The listing builds one solid part. Answer for the finished solid, in the listing's coordinates (mm). A direction names the side the tool comes from. Give positions to 0.01 mm unless a question says otherwise; leave off trailing zeros. Loops run counter-clockwise (first coordinate to the right, second up) from the corner with the lowest first, then second, coordinate; pieces in that order, holes last. Notation, with made-up numbers: (2.25, 27) - (53.25, 27) arc R27 ccw to (53.25, 44) - close; hole circle Ø1 at (38, 38). An arc over 180 degrees is marked (long way). Answer as CSV lines item,"result". Start each with the question number.
1) A cutting plane is placed at D-D (x = -38.5). Determine the outline of the cut face in (y, z), and give its area (3 significant figures).
2) For a pull along X with two mould halves and no side action, classify faces 4 (the face through (51.598, 9.86, 189.239)), 5 (the face through (-2, 0, 99)), 6 (the face through (0, 10, 105)), 7 (the face through (130, 296, 128)) as pulls with the +X half, pulls with the -X half, needs draft (parallel to the pull), parting line crosses it, or undercut.
3) A cutting plane is placed at C-C (x = 32). Determine the outline of the cut face in (y, z) (3 decimals), and give its area (3 significant figures).
4) A cutting plane is placed at B-B (z = 76). Determine the outline of the cut face in (x, y), and give its area (3 significant figures).
5) For faces 1 (the face through (-25, 280, 124)), 2 (the face through (-52.407, 9.86, 191.193)), 3 (the face through (2, 600, 99)), determine the directions among +Z, -Z, +X, -X, +Y, -Y from which every point of the face is accessible in a straight line to the end or side of a thin tool.
6) Find the intervals of material crossed by line 1 along Y through (x, z) = (63.5, 99); line 2 along X through (y, z) = (101.5, 236); line 3 along X through (y, z) = (341, 82.5), in increasing order.
7) Flat-ended cylindrical pins translate along their axes: pin 1 (4 mm diameter, centred on x = -68, y = 310.5, fed in from -Z); pin 2 (12 mm diameter, centred on x = 65, y = 374.5, fed in from +Z). Find the tip coordinate at first contact, or state that the pin passes through.
8) A cutting plane is placed at A-A (y = 449). Determine the outline of the cut face in (x, z), and give its area (3 significant figures).
```python
from build123d import *

# Parameters (mm, degrees)
F1_DEPTH = 260
F2_W     = 210
F2_H     = 110
F3_DEPTH = 225
F4_R     = 104.99999
F6_DEPTH = 600.001


# Not quite as in the source:
# - a fillet or chamfer is up to 0.001 mm smaller than in the source, because OpenCascade refuses the exact size


with BuildPart() as f1:
    # F0 (on Top) → F1 (new body)
    with BuildSketch(Plane.XY):
        Polygon((-130, 0), (0, 0), (130, 0), (130, 600), (-130, 600), align=None)
    extrude(amount=F1_DEPTH)

    # F2 (on face) → F3 (cut)
    with BuildSketch(Plane.XY.offset(260)):
        with Locations((0, 525)):
            Rectangle(F2_W, F2_H)
        with Locations((0, 225)):
            Rectangle(F2_W, F2_H)
        with Locations((0, 375)):
            Rectangle(F2_W, F2_H)
        with Locations((0, 75)):
            Rectangle(F2_W, F2_H)
    extrude(amount=-F3_DEPTH, mode=Mode.SUBTRACT)

    # F4 (radius 105 in the source; OpenCascade refuses exactly that, so slightly less here)
    f4_edges = [f1.edges().sort_by_distance(p)[0] for p in [
        (-105, 75, 35),
        (105, 75, 35),
        (-105, 225, 35),
        (-105, 375, 35),
        (-105, 525, 35),
        (105, 225, 35),
        (105, 375, 35),
        (105, 525, 35),
    ]]
    fillet(f4_edges, radius=F4_R)

    # F5 (on face) → F6 (cut, through all)
    with BuildSketch(Plane.XZ):
        with BuildLine():
            ThreePointArc((23.0969883128, 120.4329141909), (24.5196320101, 125.1227419496), (25, 130))
            ThreePointArc((25, 130), (-4.8772580504, 154.5196320101), (-23.0969883128, 120.4329141909))
            ThreePointArc((-23.0969883128, 120.4329141909), (0, 105), (23.0969883128, 120.4329141909))
        make_face()
        with BuildLine():
            ThreePointArc((-23.0969883128, 120.4329141909), (-4.8772580504, 154.5196320101), (25, 130))
            ThreePointArc((25, 130), (24.5196320101, 125.1227419496), (23.0969883128, 120.4329141909))
            Line((23.0969883128, 120.4329141909), (80.9075681158, 260))
            Line((80.9075681158, 260), (0, 260))
            Line((0, 260), (-80.9075681158, 260))
            Line((-80.9075681158, 260), (-23.0969883128, 120.4329141909))
        make_face()
    extrude(amount=-F6_DEPTH, mode=Mode.SUBTRACT)


solid = f1.part
```
Ans:
1,outline,"(0, 0) - (600, 0) - (600, 157.62) - (580, 157.62) - (580, 42.31) - (470, 42.31) - (470, 157.62) - (430, 157.62) - (430, 42.31) - (320, 42.31) - (320, 157.62) - (280, 157.62) - (280, 42.31) - (170, 42.31) - (170, 157.62) - (130, 157.62) - (130, 42.31) - (20, 42.31) - (20, 157.62) - (0, 157.62) - close"
1,area,"43,800 mm2"
2,face 4,"undercut"
2,face 5,"needs draft"
2,face 6,"undercut"
2,face 7,"pulls with the +X half"
3,outline,"(0, 0) - (600, 0) - (600, 141.927) - (580, 141.927) - (580, 39.995) - (470, 39.995) - (470, 141.927) - (430, 141.927) - (430, 39.995) - (320, 39.995) - (320, 141.927) - (280, 141.927) - (280, 39.995) - (170, 39.995) - (170, 141.927) - (130, 141.927) - (130, 39.995) - (20, 39.995) - (20, 141.927) - (0, 141.927) - close"
3,area,"40,300 mm2"
4,outline,"(-130, 0) - (130, 0) - (130, 600) - (-130, 600) - close; hole (-83.24, 20) - (83.24, 20) - (83.24, 130) - (-83.24, 130) - close; hole (-83.24, 170) - (83.24, 170) - (83.24, 280) - (-83.24, 280) - close; hole (-83.24, 320) - (83.24, 320) - (83.24, 430) - (-83.24, 430) - close; hole (-83.24, 470) - (83.24, 470) - (83.24, 580) - (-83.24, 580) - close"
4,area,"82,700 mm2"
5,face 1,"+Z"
5,face 2,"+Z, +Y, -Y"
5,face 3,"+Z, -Z, +X, -X, +Y"
6,line 1,"0 to 20, 130 to 170, 280 to 320, 430 to 470, 580 to 600"
6,line 2,"-130 to -105, 105 to 130"
6,line 3,"-130 to -87.86, 87.86 to 130"
7,pin 1,"z = 0"
7,pin 2,"z = 62.64"
8,outline,"(-130, 0) - (130, 0) - (130, 260) - (80.91, 260) - (23.1, 120.43) arc R25 cw to (-23.1, 120.43) - (-80.91, 260) - (-130, 260) - close"
8,area,"52,600 mm2"
